```python
from build123d import *

# Parameters (mm, degrees)
SKETCH1_W             = 52.07
SKETCH1_H             = 52.07
SKETCH1_W_2           = 41.91
SKETCH1_H_2           = 41.91
BOSS_EXTRUDE1_DEPTH   = 7.874
BOSS_EXTRUDE1_2_DEPTH = 7.874
BOSS_EXTRUDE3_DEPTH   = 5.08
BOSS_EXTRUDE3_2_DEPTH = 5.08
SKETCH3_W             = 52.07
SKETCH3_H             = 52.07
BOSS_EXTRUDE4_DEPTH   = 5.08


with BuildPart() as part:
    # Sketch1 → Boss-Extrude1 (new body)
    with BuildSketch(Plane.XY):
        with Locations((20.955, 20.955)):
            Rectangle(SKETCH1_W, SKETCH1_H)
        with Locations((20.955, 20.955)):
            Rectangle(SKETCH1_W_2, SKETCH1_H_2, mode=Mode.SUBTRACT)
    extrude(amount=BOSS_EXTRUDE1_DEPTH)



with BuildPart() as body_2:
    # Sketch1 → Boss-Extrude1 2 (new body)
    with BuildSketch(Plane.XY):
        with Locations((479.425, 20.955)):
            Rectangle(SKETCH1_W, SKETCH1_H)
        with Locations((479.425, 20.955)):
            Rectangle(SKETCH1_W_2, SKETCH1_H_2, mode=Mode.SUBTRACT)
    extrude(amount=BOSS_EXTRUDE1_2_DEPTH)


with BuildPart() as body_3:
    # Sketch2 → Boss-Extrude3 (new body)
    with BuildSketch(Plane(origin=(0, 0, 0), x_dir=(-1, 0, 0), z_dir=(0, 0, -1))):
        Polygon((-8.255, -132.08), (-8.255, -5.08), (-33.655, -5.08), (-33.655, -106.68), (-466.725, -106.68), (-466.725, -5.08), (-492.125, -5.08), (-492.125, -132.08), align=None)
    extrude(amount=BOSS_EXTRUDE3_DEPTH)


with BuildPart() as body_4:
    # Sketch2 → Boss-Extrude3 2 (new body)
    with BuildSketch(Plane(origin=(0, 0, 0), x_dir=(-1, 0, 0), z_dir=(0, 0, -1))):
        Polygon((-33.655, 46.99), (-8.255, 46.99), (-8.255, 173.99), (-492.125, 173.99), (-492.125, 46.99), (-466.725, 46.99), (-466.725, 148.59), (-33.655, 148.59), align=None)
    extrude(amount=BOSS_EXTRUDE3_2_DEPTH)


with BuildPart() as part_1:
    add(part.part)

    add(body_2.part)  # Boss-Extrude4 merges body 2

    add(body_3.part)  # Boss-Extrude4 merges body 3

    add(body_4.part)  # Boss-Extrude4 merges body 4
    # Sketch3 → Boss-Extrude4 (add)
    with BuildSketch(Plane(origin=(0, 0, 0), x_dir=(-1, 0, 0), z_dir=(0, 0, -1))):
        with Locations((-20.955, 20.955)):
            Rectangle(SKETCH3_W, SKETCH3_H)
        with Locations((-479.425, 20.955)):
            Rectangle(SKETCH3_W, SKETCH3_H)
    extrude(amount=BOSS_EXTRUDE4_DEPTH)


solid = part_1.part
```
Design review of the part built by this model. Coordinates are the model's own, in mm. A direction names the side the tool comes from. Coordinates: 2 decimals unless noted, no trailing zeros. Write each loop counter-clockwise with the first axis right and the second up, starting at its lowest first coordinate (ties: lowest second). Pieces come first, ordered by that corner, then holes.
1) Machinability: for faces 1 (the flat face through (453.39, 21, 1)), 2 (the flat face through (251, 158, 0)), 3 (the flat face through (254, -113, -5.08)), 4 (the flat face through (479, -5.08, 3)), which of the approach directions +Z, -Z, +X, -X, +Y, -Y give a long, thin tool a straight path to every point of the face, cutting with its end or side? Answer none if there is none.
2) Insertion check: pin 1 (2 mm diameter, centred on y = -39, z = -2.5, fed in from -X) (3 decimals); pin 2 (6.5 mm diameter, centred on x = 469, z = 5, fed in from -Y); pin 3 (1 mm diameter, centred on y = -43, z = -3, fed in from +X) (3 decimals). Each pin has a flat end and moves straight along its axis. Give the tip position at first contact, or say it passes through.
3) Add section C-C (x = 71). Write out the cut boundary in (y, z), plus the area to 3 significant figures.
4) To check wall thickness, follow L1, parallel to X at y = 6, z = 3.25; L2, parallel to X at y = -38, z = -3 (3 decimals); L3, parallel to X at y = 34.5, z = -2.25. State the ranges of each line that lie inside material, in increasing order.
5) Add section D-D (y = 142). Write out the cut boundary in (x, z) (3 decimals).
6) Add section B-B (y = 30). Write out the cut boundary in (x, z).
7) Mouldability with a two-part tool opening along X and no side actions: class faces 5 (the flat face through (505.46, 21, 1)), 6 (the flat face through (251, -115, 0)), 7 (the flat face through (46.99, 21, 1)) as +X half, -X half, draft (parallel to the pull), parting line (faces both ways), or undercut.
8) Add section A-A (z = 4). Write out the cut boundary in (x, y).
Check result:
1. face 1: +Z, -Z
1. face 2: +Z, +X, -X, +Y
1. face 3: -Z, +X, -X, +Y, -Y
1. face 4: +Z
2. pin 1: stops at x = 8.255
2. pin 2: stops at y = -5.08
2. pin 3: stops at x = 492.125
3. outline: (-132.08, -5.08) - (-106.68, -5.08) - (-106.68, 0) - (-132.08, 0) - close; (148.59, -5.08) - (173.99, -5.08) - (173.99, 0) - (148.59, 0) - close
3. area: 258 mm2
4. L1: x = -5.08 to 0, 41.91 to 46.99, 453.39 to 458.47, 500.38 to 505.46
4. L2: x = 8.255 to 33.655, 466.725 to 492.125
4. L3: x = -5.08 to 46.99, 453.39 to 505.46
5. outline: (8.255, -5.08) - (33.655, -5.08) - (33.655, 0) - (8.255, 0) - close; (466.725, -5.08) - (492.125, -5.08) - (492.125, 0) - (466.725, 0) - close
6. outline: (-5.08, -5.08) - (46.99, -5.08) - (46.99, 7.87) - (41.91, 7.87) - (41.91, 0) - (0, 0) - (0, 7.87) - (-5.08, 7.87) - close; (453.39, -5.08) - (505.46, -5.08) - (505.46, 7.87) - (500.38, 7.87) - (500.38, 0) - (458.47, 0) - (458.47, 7.87) - (453.39, 7.87) - close
7. face 5: +X half
7. face 6: draft
7. face 7: undercut
8. outline: (-5.08, -5.08) - (46.99, -5.08) - (46.99, 46.99) - (-5.08, 46.99) - close; (453.39, -5.08) - (505.46, -5.08) - (505.46, 46.99) - (453.39, 46.99) - close; hole (0, 0) - (41.91, 0) - (41.91, 41.91) - (0, 41.91) - close; hole (458.47, 0) - (500.38, 0) - (500.38, 41.91) - (458.47, 41.91) - close
